The figure shows three views and two pictorial views of one solid part (mm, origin at its lowest corner). Answer the questions. A direction names the side the tool comes from. Coordinates: 2 decimals unless noted, no trailing zeros. Write each loop counter-clockwise with the first axis right and the second up, starting at its lowest first coordinate (ties: lowest second). Pieces come first, ordered by that corner, then holes. Notation, with made-up numbers: (60, 3.25) - (116, 3.25) arc R28 cw to (116, 31.25) - close; hole circle Ø7 at (28.5, 72). An arc over 180 degrees is marked (long way). Use a Markdown table: item, result. Add a question column.
(1) The part is cut by section D-D, the plane z = 62. Give the vertices of the cut face in (x, y).
(2) The part is cut by section B-B, the plane z = 14. Give the vertices of the cut face in (x, y).
(3) The part is cut by section A-A, the plane x = 158.5. Give the vertices of the cut face in (y, z).
(4) A tool of negligible diameter and unlimited length cuts with its end or side. For the marked faces 1, 2 and 3, from which of +Z, -Z, +X, -X, +Y, -Y can it reach the whole face along a straight path? Write none if from no direction.
(5) Find the intervals of material crossed by line 1 (X direction, y = 103.5, z = 83.5); line 2 (Z direction, x = 109, y = 132); line 3 (Z direction, x = 79, y = 7), in increasing order. Write a range as from..to.
(6) Given pin 1 Ø6 at (y, z) = (54, 119) entering from +X; pin 2 Ø10 at (x, y) = (137, 50) entering from -Z; pin 3 Ø4 at (x, y) = (165.5, 110.5) entering from -Z; pin 4 Ø1.6 at (y, z) = (95, 8.5) entering from +X, each flat-ended and moving along its own axis, determine where each tip first touches the part or whether it passes through.
(7) The part is cut by section C-C, the plane y = 100. Give the vertices of the cut face in (x, z), then the cut area to 3 significant figures.
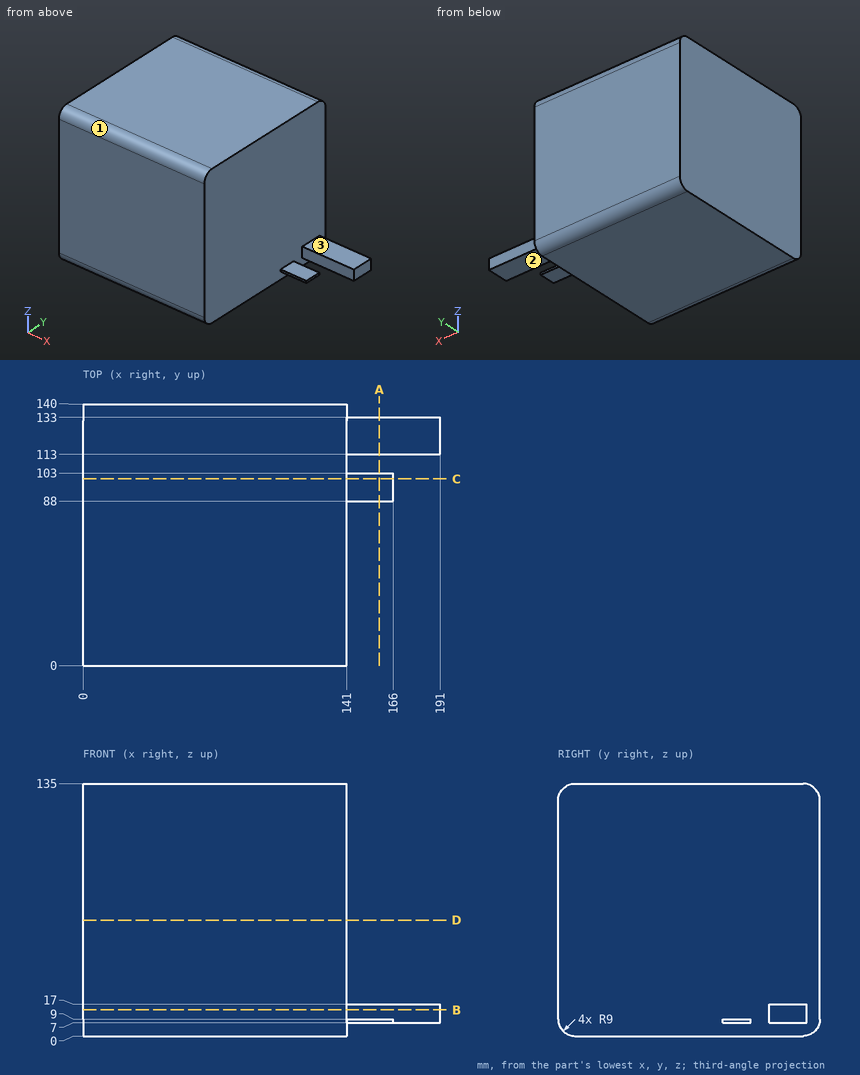
Model answer:
| question | item | result |
|---|---|---|
| 1 | outline | (0, 0) - (141, 0) - (141, 140) - (0, 140) - close |
| 2 | outline | (0, 0) - (141, 0) - (141, 113) - (191, 113) - (191, 133) - (141, 133) - (141, 140) - (0, 140) - close |
| 3 | outline | (88, 7) - (103, 7) - (103, 9) - (88, 9) - close; (113, 7) - (133, 7) - (133, 17) - (113, 17) - close |
| 4 | face 1 | +Z, +X, -X, -Y |
| 4 | face 2 | -Z, +X, +Y, -Y |
| 4 | face 3 | +Z, +X, +Y, -Y |
| 5 | line 1 | 0..141 |
| 5 | line 2 | 0.06..134.94 |
| 5 | line 3 | 0.23..134.77 |
| 6 | pin 1 | x = 141 |
| 6 | pin 2 | z = 0 |
| 6 | pin 3 | through |
| 6 | pin 4 | x = 166 |
| 7 | outline | (0, 0) - (141, 0) - (141, 7) - (166, 7) - (166, 9) - (141, 9) - (141, 135) - (0, 135) - close |
| 7 | area | 19,100 mm^2 |
